Input: part model. Units: mm. Frame: model coordinates. Give positions to 0.01 mm unless a question says otherwise; leave off trailing zeros. Loops run counter-clockwise (first coordinate to the right, second up) from the corner with the lowest first, then second, coordinate; pieces in that order, holes last.
from build123d import *

# Parameters (mm, degrees)
SKETCH1_R           = 1
BOSS_EXTRUDE1_DEPTH = 0.5


with BuildPart() as part:
    # Sketch1 → Boss-Extrude1 (new, symmetric)
    with BuildSketch(Plane.XY):
        with BuildLine():
            Line((6.085309509, 5.469141511), (-5.830437798, -0.839652689))
            ThreePointArc((-5.830437798, -0.839652689), (-6.333032181, -1.964493074), (-5.362523581, -2.723426577))
            Line((-5.362523581, -2.723426577), (29.297564453, -2.723426577))
            ThreePointArc((29.297564453, -2.723426577), (30.288426963, -1.858302391), (29.56485123, -0.759809547))
            Line((29.56485123, -0.759809547), (6.820510503, 5.548984653))
            ThreePointArc((6.820510503, 5.548984653), (6.44525811, 5.579522252), (6.085309509, 5.469141511))
        make_face()
        with Locations((6.611324324, 4.050373423)):
            Circle(SKETCH1_R, mode=Mode.SUBTRACT)
        with Locations((-3.349575676, -1.223426577)):
            Circle(SKETCH1_R, mode=Mode.SUBTRACT)
        with Locations((25.624324324, -1.223426577)):
            Circle(SKETCH1_R, mode=Mode.SUBTRACT)
    extrude(amount=BOSS_EXTRUDE1_DEPTH, both=True)


solid = part.part
(1) Cut plane C-C (y = 1.5). Return the cut outline in (x, z), and give its area (3 significant figures).
Values follow:
outline: (-1.41, -0.5) - (21.42, -0.5) - (21.42, 0.5) - (-1.41, 0.5) - close
area: 22.8 mm2
(2) Ray query, probe 1 along X at (y, z) = (-1.75, -0.25); probe 2 along X at (y, z) = (-2, 0.2); probe 3 along Y at (x, z) = (-2.5, 0.25). Return the intervals inside material, ascending.
Values follow:
probe 1: x = -6.36 to -4.2, -2.5 to 24.77, 26.47 to 30.3
probe 2: x = -6.32 to -3.98, -2.72 to 24.99, 26.25 to 30.26
probe 3: y = -2.72 to -1.75, -0.7 to 0.92
(3) Mould query, pull axis X, two halves, no side actions, for faces 1 (the cylindrical face through (30.286, -1.878, 0.007)), 2 (the flat face through (12, 1, -0.5)), 3 (the cylindrical face through (26.548, -1.606, -0.007)). Classes: +X half, -X half, draft (parallel to the pull), parting line (faces both ways), or undercut.
Values follow:
face 1: +X half
face 2: draft
face 3: undercut
(4) Cut plane B-B (x = 20.5). Return the cut outline in (y, z), and give its area (3 significant figures).
Values follow:
outline: (-2.72, -0.5) - (1.75, -0.5) - (1.75, 0.5) - (-2.72, 0.5) - close
area: 4.48 mm2
(5) Pin query (flat end, axial travel): pin 1 Ø1.2 at (x, y) = (6.61, 4.05) entering from -Z. Return the tip coordinate at first contact, or that it passes through.
Values follow:
pin 1: passes through
(6) Cut plane A-A (z = 0.1). Return the cut outline in (x, y), and give its area (3 significant figures).
Values follow:
outline: (-5.83, -0.84) arc R1 ccw to (-5.36, -2.72) - (29.3, -2.72) arc R1 ccw to (29.56, -0.76) - (6.82, 5.55) arc R1 ccw to (6.09, 5.47) - close; hole circle Ø2 at (-3.35, -1.22); hole circle Ø2 at (6.61, 4.05); hole circle Ø2 at (25.62, -1.22)
area: 175 mm2
